Work out the finished part from the listing and answer in its coordinate system (mm). A direction names the side the tool comes from. Coordinates: 2 decimals unless noted, no trailing zeros. Order: outer loops, then holes, each group sorted by start corner. A loop starts at its lowest first (then second) coordinate and runs counter-clockwise, first axis right, second up. Notation, with made-up numbers: (5, 85.5) - (56, 85.5) arc R14 ccw to (56, 99.5) - close; hole circle Ø6 at (-24.5, -23.5). An arc over 180 degrees is marked (long way). Answer as a JSON object with one key per item and string values. Group by question number.
1) Find the intervals of material crossed by line 1 along Y through (x, z) = (44, 19.75); line 2 along X through (y, z) = (8, 8); line 3 along Y through (x, z) = (-22, 12.5), in increasing order.
2) Section D-D (x = -2.5) is taken. Give the vertices of the cut face in (y, z).
3) Each of these flat-tipped pins is pushed along its axis until it touches: P1, Ø1.5, axis at y = 23.5, z = 5, coming from the +X side (3 decimals); P2, Ø4, axis at x = 12.7, y = -25.4, coming from the -Z side; P3, Ø4, axis at x = 13.5, y = -15, coming from the +Z side. Where does it stop, or does it pass through?
4) Section A-A (z = 18) is taken. Count the separate pieces of the cut face and the enclosed holes in it, plus the area to 3 significant figures.
5) The mould has two halves that part along X. Classify faces 3 (the face through (-59.68, 34.48, 12.52)), 4 (the face through (56.25, -23.68, 14.13)), 5 (the face through (-13.11, 28.55, 12.88)), 6 (the face through (-35.6, 22.9, 25.4)): released by +X, released by -X, zero draft, split by the parting line, or undercut.
6) A tool of negligible diameter and unlimited length cuts with its end or side. For faces 1 (the face through (0, 35.56, 14)), 2 (the face through (-48, 23, 25.4)), from which of +Z, -Z, +X, -X, +Y, -Y can it reach the whole face along a straight path? Write none if from no direction.
from build123d import *

# Parameters (mm, degrees)
F1_DEPTH = 25.4
F3_R     = 3.175
F4_DEPTH = 25.4
F5_T     = -2.54


with BuildPart() as f1:
    # F0 (on Top) → F1 (new body)
    with BuildSketch(Plane.XY):
        with BuildLine():
            Line((50.8, 38.1), (-50.8, 38.1))
            ThreePointArc((-50.8, 38.1), (-59.780256, 34.380256), (-63.5, 25.4))
            Line((-63.5, 25.4), (-63.5, -38.1))
            Line((-63.5, -38.1), (63.5, -38.1))
            Line((63.5, -38.1), (63.5, 12.7))
            Line((63.5, 12.7), (50.8, 38.1))
        make_face()
    extrude(amount=F1_DEPTH)

    # F3 (on face) → F4 (cut)
    with BuildSketch(Plane.XY.offset(25.4)):
        with Locations((-50.8, 25.4)):
            Circle(F3_R)
        with Locations((-50.8, 0)):
            Circle(F3_R)
        with Locations((-50.8, -25.4)):
            Circle(F3_R)
        with Locations((-38.1, 25.4)):
            Circle(F3_R)
        with Locations((-38.1, 0)):
            Circle(F3_R)
        with Locations((-38.1, -25.4)):
            Circle(F3_R)
        with Locations((-25.4, 25.4)):
            Circle(F3_R)
        with Locations((-25.4, 0)):
            Circle(F3_R)
        with Locations((-25.4, -25.4)):
            Circle(F3_R)
        with Locations((-12.7, 25.4)):
            Circle(F3_R)
        with Locations((-12.7, 0)):
            Circle(F3_R)
        with Locations((-12.7, -25.4)):
            Circle(F3_R)
        with Locations((50.8, 25.4)):
            Circle(F3_R)
        with Locations((38.1, 25.4)):
            Circle(F3_R)
        with Locations((25.4, 25.4)):
            Circle(F3_R)
        with Locations((12.7, 25.4)):
            Circle(F3_R)
        with Locations((12.7, 0)):
            Circle(F3_R)
        with Locations((25.4, 0)):
            Circle(F3_R)
        with Locations((38.1, 0)):
            Circle(F3_R)
        with Locations((50.8, -25.4)):
            Circle(F3_R)
        with Locations((38.1, -25.4)):
            Circle(F3_R)
        with Locations((25.4, -25.4)):
            Circle(F3_R)
        with Locations((12.7, -25.4)):
            Circle(F3_R)
        with Locations((50.8, 0)):
            Circle(F3_R)
    extrude(amount=-F4_DEPTH, mode=Mode.SUBTRACT)

    # F5
    f5_openings = [f1.faces().sort_by_distance(p)[0] for p in [
        (-0.855292, -0.687975, 25.4),
    ]]
    offset(amount=F5_T, openings=f5_openings)


solid = f1.part
Report:
{
 "1": {"line 1": "y = -38.1 to -35.56, 35.56 to 38.1", "line 2": "x = -63.5 to -60.96, 60.96 to 63.5", "line 3": "y = -38.1 to -35.56, -29.99 to -20.81, -4.59 to 4.59, 20.81 to 29.99, 35.56 to 38.1"},
 "2": {"outline": "(-38.1, 0) - (38.1, 0) - (38.1, 25.4) - (35.56, 25.4) - (35.56, 2.54) - (-35.56, 2.54) - (-35.56, 25.4) - (-38.1, 25.4) - close"},
 "3": {"P1": "stops at x = 58.475", "P2": "passes through", "P3": "stops at z = 2.54"},
 "4": {"separate pieces": "24", "enclosed holes": "25", "area": "2,660 mm²"},
 "5": {"face 3": "released by -X", "face 4": "undercut", "face 5": "undercut", "face 6": "zero draft"},
 "6": {"face 1": "+Z", "face 2": "+Z, +X, -X, +Y, -Y"}
}
